from build123d import *

# Parameters (mm, degrees)
F0_W     = 63.5
F0_H     = 19.05
F1_DEPTH = 31.75
F2_T     = -1.3208
F3_R     = 5.9944
F3_R_2   = 4.6736
F4_DEPTH = 5.08
F5_R     = 1.27


with BuildPart() as f1:
    # F0 (on Top) → F1 (new body)
    with BuildSketch(Plane.XY):
        with Locations((-31.75, 9.525)):
            Rectangle(F0_W, F0_H)
    extrude(amount=F1_DEPTH)

    # F2
    f2_openings = [f1.faces().sort_by_distance(p)[0] for p in [
        (-31.75, 0, 15.875),
    ]]
    offset(amount=F2_T, openings=f2_openings)

    # F3 (on face) → F4 (join)
    with BuildSketch(Plane(origin=(0, 19.05, 0), x_dir=(-1, 0, 0), z_dir=(0, 1, 0))):
        with Locations((7.874, 23.876)):
            Circle(F3_R)
        with Locations((7.874, 23.876)):
            Circle(F3_R_2, mode=Mode.SUBTRACT)
        with Locations((23.876, 23.876)):
            Circle(F3_R)
        with Locations((23.876, 23.876)):
            Circle(F3_R_2, mode=Mode.SUBTRACT)
        with Locations((39.878, 23.876)):
            Circle(F3_R)
        with Locations((39.878, 23.876)):
            Circle(F3_R_2, mode=Mode.SUBTRACT)
        with Locations((55.88, 23.876)):
            Circle(F3_R)
        with Locations((55.88, 23.876)):
            Circle(F3_R_2, mode=Mode.SUBTRACT)
        with Locations((8.275095, 7.751988)):
            Circle(F3_R)
        with Locations((8.275095, 7.751988)):
            Circle(F3_R_2, mode=Mode.SUBTRACT)
        with Locations((56.281095, 7.751988)):
            Circle(F3_R)
        with Locations((56.281095, 7.751988)):
            Circle(F3_R_2, mode=Mode.SUBTRACT)
        with Locations((40.279095, 7.751988)):
            Circle(F3_R)
        with Locations((40.279095, 7.751988)):
            Circle(F3_R_2, mode=Mode.SUBTRACT)
        with Locations((24.277095, 7.751988)):
            Circle(F3_R)
        with Locations((24.277095, 7.751988)):
            Circle(F3_R_2, mode=Mode.SUBTRACT)
    extrude(amount=F4_DEPTH)

    # F5
    f5_edges = [f1.edges().sort_by_distance(p)[0] for p in [
        (-31.75, 19.05, 31.75),
        (-63.5, 9.525, 31.75),
        (-31.75, 0, 31.75),
        (0, 9.525, 31.75),
        (-63.5, 19.05, 15.875),
        (-63.5, 0, 15.875),
        (-63.5, 9.525, 0),
        (0, 0, 15.875),
        (0, 19.05, 15.875),
        (0, 9.525, 0),
        (-31.75, 19.05, 0),
        (-31.75, 0, 0),
    ]]
    fillet(f5_edges, radius=F5_R)


solid = f1.part
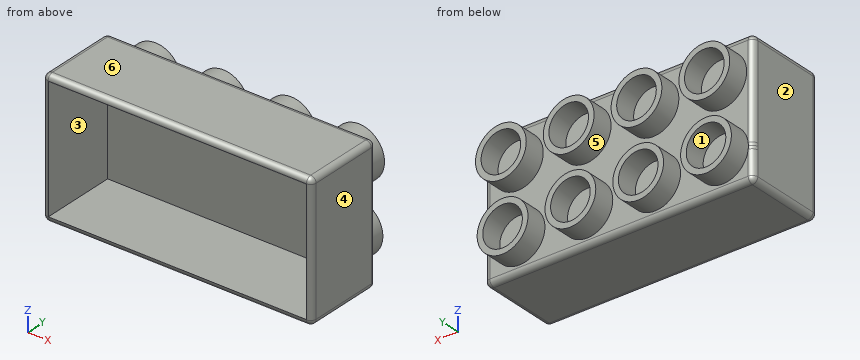
Check sheet for the modelled part. Datum: model origin and axes. Units: mm. Face numbers are marked on the shaded views. A direction names the side the tool comes from. Round coordinates to 2 decimals unless told otherwise and drop trailing zeros. Write each loop counter-clockwise with the first axis right and the second up, starting at its lowest first coordinate (ties: lowest second). Pieces come first, ordered by that corner, then holes. Notation, with made-up numbers: (-31, -13) - (-1, -13) arc R4 ccw to (-1, -9) - close; hole circle Ø6 at (-22, 12). An arc over 180 degrees is marked (long way). Return JSON: item names as keys, results as strings.
Q1. Depth check by flat-ended pin: P1, Ø2, axis at x = -49, z = 26, coming from the -Y side; P2, Ø12, axis at x = -56.28, z = 7.75, coming from the -Y side; P3, Ø4.5, axis at x = -8.5, z = 24.5, coming from the +Y side; P4, Ø6, axis at y = 21, z = 16.5, coming from the +X side. Enter the tip coordinate at first touch or a pass-through.
Returned:
{"P1": "stops at y = 17.73", "P2": "stops at y = 0", "P3": "stops at y = 19.05", "P4": "stops at x = -0.02"}
Q2. Cross-section at A-A (y = 3.5). Record the boundary of the cut face in (x, z).
Returned:
{"outline": "(-63.5, 1.27) arc R1.27 ccw to (-62.23, 0) - (-1.27, 0) arc R1.27 ccw to (0, 1.27) - (0, 30.48) arc R1.27 ccw to (-1.27, 31.75) - (-62.23, 31.75) arc R1.27 ccw to (-63.5, 30.48) - close; hole (-62.18, 1.32) - (-1.32, 1.32) - (-1.32, 30.43) - (-62.18, 30.43) - close"}
Q3. Cross-section at B-B (x = -15). Record the boundary of the cut face in (y, z), then the cut area to 3 significant figures.
Returned:
{"outline": "(0, 1.27) arc R1.27 ccw to (1.27, 0) - (17.78, 0) arc R1.27 ccw to (19.05, 1.27) - (19.05, 30.48) arc R1.27 ccw to (17.78, 31.75) - (1.27, 31.75) arc R1.27 ccw to (0, 30.48) - (0, 30.43) - (17.73, 30.43) - (17.73, 1.32) - (0, 1.32) - close", "area": "87.4 mm²"}
Q4. Cross-section at C-C (x = -7.5). Record the boundary of the cut face in (y, z), then the cut area to 3 significant figures.
Returned:
{"outline": "(0, 1.27) arc R1.27 ccw to (1.27, 0) - (17.78, 0) arc R1.27 ccw to (19.05, 1.27) - (19.05, 1.81) - (24.13, 1.81) - (24.13, 3.14) - (19.05, 3.14) - (19.05, 12.36) - (24.13, 12.36) - (24.13, 13.7) - (19.05, 13.7) - (19.05, 17.89) - (24.13, 17.89) - (24.13, 19.22) - (19.05, 19.22) - (19.05, 28.53) - (24.13, 28.53) - (24.13, 29.86) - (19.05, 29.86) - (19.05, 30.48) arc R1.27 ccw to (17.78, 31.75) - (1.27, 31.75) arc R1.27 ccw to (0, 30.48) - (0, 30.43) - (17.73, 30.43) - (17.73, 1.32) - (0, 1.32) - close", "area": "114 mm²"}
Q5. Access from +Z, -Z, +X, -X, +Y, -Y to the whole of each face (thin tool, end or side, straight path). Record for the marked faces 1, 2 and 3.
Returned:
{"face 1": "+Y", "face 2": "+Z, -Z, -X, +Y, -Y", "face 3": "-Y"}
Q6. Cross-section at D-D (x = -55.88). Record the boundary of the cut face in (y, z), then the cut area to 3 significant figures.
Returned:
{"outline": "(0, 1.27) arc R1.27 ccw to (1.27, 0) - (17.78, 0) arc R1.27 ccw to (19.05, 1.27) - (19.05, 1.77) - (24.13, 1.77) - (24.13, 3.1) - (19.05, 3.1) - (19.05, 12.41) - (24.13, 12.41) - (24.13, 13.73) - (19.05, 13.73) - (19.05, 17.88) - (24.13, 17.88) - (24.13, 19.2) - (19.05, 19.2) - (19.05, 28.55) - (24.13, 28.55) - (24.13, 29.87) - (19.05, 29.87) - (19.05, 30.48) arc R1.27 ccw to (17.78, 31.75) - (1.27, 31.75) arc R1.27 ccw to (0, 30.48) - (0, 30.43) - (17.73, 30.43) - (17.73, 1.32) - (0, 1.32) - close", "area": "114 mm²"}
Q7. Draft check along X on the marked faces 4, 5 and 6. Enter one of: released by +X, released by -X, zero draft, split by the parting line, or undercut.
Returned:
{"face 4": "released by +X", "face 5": "undercut", "face 6": "zero draft"}
Q8. Scan lines: L1, parallel to X at y = 2.25, z = 13; L2, parallel to Z at x = -55.88, y = 21.3; L3, parallel to Z at x = -54.5, y = 14. Record each from-to range of solid material in increasing order. Write a range as from..to.
Returned:
{"L1": "x = -63.5..-62.18, -1.32..0", "L2": "z = 1.77..3.1, 12.41..13.73, 17.88..19.2, 28.55..29.87", "L3": "z = 0..1.32, 30.43..31.75"}
